The listing builds one solid part. Answer for the finished solid, in the listing's coordinates (mm). Face numbers are marked on the shaded views. A direction names the side the tool comes from. Coordinates: 2 decimals unless noted, no trailing zeros. Loops run counter-clockwise (first coordinate to the right, second up) from the corner with the lowest first, then second, coordinate; pieces in that order, holes last. Notation, with made-up numbers: (6, 69.25) - (48, 69.25) arc R21 cw to (48, 74.25) - close; hole circle Ø1 at (-27.75, -40). An arc over 180 degrees is marked (long way). One line per question, with ' | ' between items.
from build123d import *

# Parameters (mm, degrees)
F0_R     = 3.302
F1_DEPTH = 101.6
F2_R     = 3.302
F3_DEPTH = 16.35888
F4_W     = 38.1
F4_H     = 33.4236365795
F4_R     = 4.7625
F5_DEPTH = 58.56755
F6_R     = 9.525
F7_DEPTH = 31.751


with BuildPart() as f1:
    # F0 (on Front) → F1 (new body)
    with BuildSketch(Plane.XZ):
        with BuildLine():
            Line((0, 0), (6.35, 0))
            ThreePointArc((6.35, 0), (8.2098719395, 4.4901280605), (12.7, 6.35))
            Line((12.7, 6.35), (52.324, 6.35))
            ThreePointArc((52.324, 6.35), (56.8141280605, 4.4901280605), (58.674, 0))
            Line((58.674, 0), (65.024, 0))
            Line((65.024, 0), (65.024, 31.75))
            Line((65.024, 31.75), (50.8, 31.75))
            Line((50.8, 31.75), (50.8, 38.1))
            Line((50.8, 38.1), (57.912, 38.1))
            Line((57.912, 38.1), (57.912, 65.1736365795))
            Line((57.912, 65.1736365795), (51.562, 65.1736365795))
            Line((51.562, 65.1736365795), (35.814, 49.4256365795))
            Line((35.814, 49.4256365795), (35.814, 43.0756365795))
            Line((35.814, 43.0756365795), (29.21, 43.0756365795))
            Line((29.21, 43.0756365795), (29.21, 49.4256365795))
            Line((29.21, 49.4256365795), (13.462, 65.1736365795))
            Line((13.462, 65.1736365795), (7.112, 65.1736365795))
            Line((7.112, 65.1736365795), (7.112, 38.1))
            Line((7.112, 38.1), (14.224, 38.1))
            Line((14.224, 38.1), (14.224, 31.75))
            Line((14.224, 31.75), (0, 31.75))
            Line((0, 31.75), (0, 0))
        make_face()
        with Locations((32.512, 22.225)):
            Circle(F0_R, mode=Mode.SUBTRACT)
        with Locations((32.512, 22.225)):
            Circle(F0_R)
    extrude(amount=F1_DEPTH)

    # F2 (on face) → F3 (cut)
    with BuildSketch(Plane.XZ.offset(101.6)):
        with Locations((32.512, 22.225)):
            Circle(F2_R)
    extrude(amount=-F3_DEPTH, mode=Mode.SUBTRACT)

    # F4 (on Right) → F5 (cut)
    with BuildSketch(Plane.YZ):
        with Locations((-50.8, 48.4618182898)):
            Rectangle(F4_W, F4_H)
        with Locations((-50.8, 15.875)):
            Circle(F4_R)
    extrude(amount=F5_DEPTH, mode=Mode.SUBTRACT)

    # F6 (on face) → F7 (cut, through all)
    with BuildSketch(Plane.XY.offset(31.75)):
        with Locations((32.512, -50.8)):
            Circle(F6_R)
    extrude(amount=-F7_DEPTH, mode=Mode.SUBTRACT)


solid = f1.part
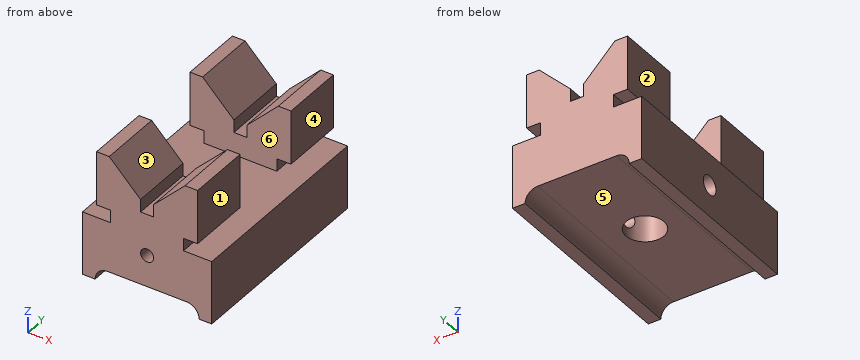
Item 1: Find the intervals of material crossed by line 1 (Y direction, x = 23, z = 46); line 2 (X direction, y = -50.8, z = 24.25); line 3 (X direction, y = -80.5, z = 33.5), in increasing order. Write a range as [from, to].
Taken from the geometry:
line 1: y = [-101.6, -69.85], [-31.75, 0] | line 2: x = [0, 22.99], [42.04, 65.02] | line 3: x = [14.22, 50.8]
Item 2: Find section A-A, the plane y = -50.8. Write down the section's boundary in (x, z).
Taken from the geometry:
outline: (0, 0) - (6.35, 0) arc R6.35 cw to (12.7, 6.35) - (22.99, 6.35) - (22.99, 11.11) - (0, 11.11) - close; (0, 20.64) - (22.99, 20.64) - (22.99, 31.75) - (0, 31.75) - close; (42.04, 6.35) - (52.32, 6.35) arc R6.35 cw to (58.67, 0) - (65.02, 0) - (65.02, 31.75) - (42.04, 31.75) - (42.04, 20.64) - (58.57, 20.64) - (58.57, 11.11) - (42.04, 11.11) - close
Item 3: The mould has two halves that part along X. Classify the marked faces 1, 2 and 3: pulls with the +X half, pulls with the -X half, needs draft (parallel to the pull), parting line crosses it, or undercut.
Taken from the geometry:
face 1: pulls with the +X half | face 2: pulls with the -X half | face 3: undercut
Item 4: Each of these flat-tipped pins is pushed along its axis until it touches: pin 1 Ø5 at (y, z) = (-20.5, 36.5) entering from +X; pin 2 Ø11.5 at (x, y) = (32.512, -50.8) entering from -Z; pin 3 Ø13.5 at (y, z) = (-78, 48) entering from -X; pin 4 Ø12 at (x, y) = (28, -66.5) entering from -Z. Where does it stop, or does it pass through?
Taken from the geometry:
pin 1: stops at x = 57.91 | pin 2: passes through | pin 3: stops at x = 7.11 | pin 4: stops at z = 6.35
Item 5: Find section D-D, the plane y = -61.5. Write down the section's boundary in (x, z).
Taken from the geometry:
outline: (0, 0) - (6.35, 0) arc R6.35 cw to (12.7, 6.35) - (52.32, 6.35) arc R6.35 cw to (58.67, 0) - (65.02, 0) - (65.02, 31.75) - (0, 31.75) - close
Item 6: Find section B-B, the plane z = 54. Write down the section's boundary in (x, y).
Taken from the geometry:
outline: (7.11, -101.6) - (24.64, -101.6) - (24.64, -69.85) - (7.11, -69.85) - close; (7.11, -31.75) - (24.64, -31.75) - (24.64, 0) - (7.11, 0) - close; (40.39, -101.6) - (57.91, -101.6) - (57.91, -69.85) - (40.39, -69.85) - close; (40.39, -31.75) - (57.91, -31.75) - (57.91, 0) - (40.39, 0) - close
Item 7: Find section C-C, the plane x = 32.5. Write down the section's boundary in (y, z) (3 decimals).
Taken from the geometry:
outline: (-101.6, 6.35) - (-60.325, 6.35) - (-60.325, 31.75) - (-69.85, 31.75) - (-69.85, 43.076) - (-101.6, 43.076) - (-101.6, 25.527) - (-85.241, 25.527) - (-85.241, 18.923) - (-101.6, 18.923) - close; (-41.275, 6.35) - (0, 6.35) - (0, 43.076) - (-31.75, 43.076) - (-31.75, 31.75) - (-41.275, 31.75) - close
Item 8: Which of the six approach directions +Z, -Z, +X, -X, +Y, -Y give full straight-line access (tool end or side, diameter ignored) to the marked faces 4, 5 and 6?
Taken from the geometry:
face 4: +Z, +X, +Y, -Y | face 5: -Z, +Y, -Y | face 6: +Z, +X, -X
